Geometry check sheet. Reference: the model listing, model coordinates, mm. A direction names the side the tool comes from. Round coordinates to 2 decimals unless told otherwise and drop trailing zeros. Order: outer loops, then holes, each group sorted by start corner. A loop starts at its lowest first (then second) coordinate and runs counter-clockwise, first axis right, second up. Notation, with made-up numbers: M 56.25,83.5 L 61.25,83.5 A18 cw 61.25,93.5 Z; hole C 74,20.25 d1. An arc over 180 degrees is marked long. Return JSON: item names as keys, results as strings. Group by question number.
```python
from build123d import *

# Parameters (mm, degrees)
SKETCH_6_R          = 4.5
EXTRUDE_4_DEPTH     = 3
SKETCH_7_R          = 3.15
CUT_EXTRUDE_4_DEPTH = 2
SKETCH_8_R          = 4
EXTRUDE_5_DEPTH     = 2
EXTRUDE_7_DEPTH     = 2
EXTRUDE_8_REACH     = 10
SKETCH_11_R         = 1.65
CUT_EXTRUDE_6_DEPTH = 2
CUT_EXTRUDE_7_REACH = 9
FILLET_4_R          = 2
FILLET_1_R          = 0.3
FILLET_2_R          = 0.3
FILLET_3_R          = 0.3


with BuildPart() as part:
    # Sketch 6 → Extrude 4 (new body)
    with BuildSketch(Plane(origin=(0, 0, 0), x_dir=(1, 0, 0), z_dir=(0, 1, 0))):
        Circle(SKETCH_6_R)
    extrude(amount=-EXTRUDE_4_DEPTH)

    # Sketch 7 → Cut-Extrude 4 (cut)
    with BuildSketch(Plane(origin=(0, 0, 0), x_dir=(1, 0, 0), z_dir=(0, 1, 0))):
        Circle(SKETCH_7_R)
    extrude(amount=-CUT_EXTRUDE_4_DEPTH, mode=Mode.SUBTRACT)

    # Sketch 15 → Cut-Revolve 2 (revolve, cut)
    with BuildSketch(Plane(origin=(0, 0, 0), x_dir=(0, 0, -1), z_dir=(1, 0, 0))):
        Polygon((4.5, -3), (4.5, -2), (3.5, -3), align=None)
    revolve(axis=Axis((0, 0, 0), (0, -1, 0)), mode=Mode.SUBTRACT)



with BuildPart() as body_2:
    # Sketch 8 → Extrude 5 (new body)
    with BuildSketch(Plane(origin=(-0.5, 0, 0), x_dir=(0, 0, -1), z_dir=(1, 0, 0))):
        with Locations((-14, 2.5)):
            Circle(SKETCH_8_R)
    extrude(amount=-EXTRUDE_5_DEPTH)


with BuildPart() as part_1:
    add(part.part)

    add(body_2.part)  # Extrude 7 merges body 2
    # Sketch 9 → Extrude 7 (add)
    with BuildSketch(Plane(origin=(-0.5, 0, 0), x_dir=(0, 0, -1), z_dir=(1, 0, 0))):
        Polygon((-9.5, -3), (-15.133083988, -1.336159626), (-10.74928321, 0.169154585), (-10, 2.5), (-6.344746865, 2.002637663), (-3.5, 0), (-3.5, -3), (-3.52896076, -3), align=None)
    extrude(amount=-EXTRUDE_7_DEPTH)

    # Sketch 16 → Extrude 8 (add, up to next)
    with BuildSketch(Plane(origin=(0, 0, 3.5), x_dir=(-1, 0, 0), z_dir=(0, 0, -1)), mode=Mode.PRIVATE) as extrude_8_sk1:
        Polygon((2.5, -3), (2.5, -2.198837366), (0.5, -2.955716811), (0.5, -3), align=None)
    extrude_8_tool1 = extrude(extrude_8_sk1.sketch, amount=EXTRUDE_8_REACH, mode=Mode.PRIVATE) - part_1.part
    add(extrude_8_tool1.solids().sort_by_distance((-1.798414, -2.732173, 3.5))[0])

    # Sketch 11 → Cut-Extrude 6 (cut)
    with BuildSketch(Plane(origin=(-0.5, 0, 0), x_dir=(0, 0, -1), z_dir=(1, 0, 0))):
        with Locations((-14, 2.5)):
            Circle(SKETCH_11_R)
    extrude(amount=-CUT_EXTRUDE_6_DEPTH, mode=Mode.SUBTRACT)

    # Sketch 12 → Cut-Extrude 7 (cut, up to next)
    with BuildSketch(Plane.ZY.offset(2.5), mode=Mode.PRIVATE) as cut_extrude_7_sk1:
        Polygon((3.5, 0), (3.741657387, 0), (10, 0), (10, 2.5), (6.344746865, 2.002637663), align=None)
    cut_extrude_7_tool1 = extrude(cut_extrude_7_sk1.sketch, amount=-CUT_EXTRUDE_7_REACH, mode=Mode.PRIVATE) & part_1.part
    add(cut_extrude_7_tool1.solids().sort_by_distance((-2.5, 1.011261, 7.508576))[0], mode=Mode.SUBTRACT)

    # Fillet 4
    fillet_4_edges = [part_1.edges().sort_by_distance(p)[0] for p in [
        (-1.5, 0, 10),
    ]]
    fillet(fillet_4_edges, radius=FILLET_4_R)

    # Fillet 1
    fillet_1_edges = [part_1.edges().sort_by_distance(p)[0] for p in [
        (-3.15, 0, 0),
    ]]
    fillet(fillet_1_edges, radius=FILLET_1_R)

    # Fillet 2
    fillet_2_edges = [part_1.edges().sort_by_distance(p)[0] for p in [
        (-0.5, 2.5, 15.65),
    ]]
    fillet(fillet_2_edges, radius=FILLET_2_R)

    # Fillet 3
    fillet_3_edges = [part_1.edges().sort_by_distance(p)[0] for p in [
        (-2.5, 2.5, 15.65),
    ]]
    fillet(fillet_3_edges, radius=FILLET_3_R)


solid = part_1.part
```
Q1. Release check for a two-part mould opening along Z. For faces 4 (the face through (-0.5, 1, 12)), 5 (the face through (-1.49, 0.6, 9.43)), 6 (the face through (-2.5, -1.138, 1.917)) record: +Z half, -Z half, draft (parallel to the pull), parting line (faces both ways), or undercut.
Q2. Section check D-D on y = 5.25. Record the cut outline in (x, z).
Q3. Section check A-A on z = 0. Record the cut outline in (x, y).
Q4. Material ranges on line 1 along Z through (x, y) = (0, -1.4); line 2 along X through (y, z) = (3, 17.25), recorded low to high.
Q5. Section check B-B on x = 0. Record the cut outline in (y, z).
Q6. Section check C-C on z = 14. Record the cut outline in (x, y), plus the area to 3 significant figures.
Q7. Depth check by flat-ended pin: pin 1 Ø3 at (y, z) = (3, 6.5) entering from +X; pin 2 Ø3 at (x, z) = (0.5, 0.5) entering from +Y; pin 3 Ø5 at (y, z) = (0, 13.5) entering from -X; pin 4 Ø5 at (y, z) = (5.5, 10.5) entering from +X. Enter the tip coordinate at first touch or a pass-through.
Q8. Set-up check for faces 1 (the face through (-2, 0, 3)), 2 (the face through (-1.49, 5.78, 16.29)), 3 (the face through (0, -2, 0)): record each of +Z, -Z, +X, -X, +Y, -Y from which the full face is reachable in a straight line by a thin tool's end or side.
Geometry check:
{
 "1": {"face 4": "draft", "face 5": "-Z half", "face 6": "undercut"},
 "2": {"outline": "M -2.5,11.1 L -0.5,11.1 L -0.5,16.9 L -2.5,16.9 Z"},
 "3": {"outline": "M -4.5,-2 L -3.5,-3 L 3.5,-3 L 4.5,-2 L 4.5,0 L 3.45,0 A0.3 ccw 3.15,-0.3 L 3.15,-2 L -3.15,-2 L -3.15,-0.3 A0.3 ccw -3.45,0 L -4.5,0 Z"},
 "4": {"line 1": "z = -4.5 to -3.15, 3.15 to 4.5", "line 2": "x = -2.5 to -0.5"},
 "5": {"outline": "M -3,-3.5 L -2,-4.5 L 0,-4.5 L 0,-3.45 A0.3 ccw -0.3,-3.15 L -2,-3.15 L -2,3.15 L -0.3,3.15 A0.3 ccw 0,3.45 L 0,4.5 L -2,4.5 L -3,3.5 Z"},
 "6": {"outline": "M -2.5,-1.67 L -0.5,-1.67 L -0.5,0.55 A0.3 ccw -0.8,0.85 L -2.2,0.85 A0.3 ccw -2.5,0.55 Z; M -2.5,4.45 A0.3 ccw -2.2,4.15 L -0.8,4.15 A0.3 ccw -0.5,4.45 L -0.5,6.5 L -2.5,6.5 Z", "area": "9.66 mm^2"},
 "7": {"pin 1": "passes through", "pin 2": "stops at y = -2", "pin 3": "stops at x = -2.5", "pin 4": "stops at x = -0.5"},
 "8": {"face 1": "-Z, +X, -X, +Y", "face 2": "+X, -X", "face 3": "+Y"}
}
